from build123d import *

# Parameters (mm, degrees)
SKETCH1_W           = 300
SKETCH1_H           = 500
BOSS_EXTRUDE1_DEPTH = 20
SKETCH1_3_W         = 65
SKETCH1_3_H         = 500
BOSS_EXTRUDE2_DEPTH = 70
CUT_EXTRUDE1_START  = 70
CUT_EXTRUDE1_DEPTH  = 47


with BuildPart() as part:
    # Sketch1 → Boss-Extrude1 (new body)
    with BuildSketch(Plane.XY):
        Rectangle(SKETCH1_W, SKETCH1_H)
    extrude(amount=BOSS_EXTRUDE1_DEPTH)

    # Sketch1<3> → Boss-Extrude2 (add)
    with BuildSketch(Plane.XY):
        with Locations((182.5, 0)):
            Rectangle(SKETCH1_3_W, SKETCH1_3_H)
        with Locations((-182.5, 0)):
            Rectangle(SKETCH1_3_W, SKETCH1_3_H)
    extrude(amount=BOSS_EXTRUDE2_DEPTH)

    # Sketch1<5> → Cut-Extrude1 (cut)
    with BuildSketch(Plane.XY.offset(CUT_EXTRUDE1_START)):
        with BuildLine():
            Line((-164.5, 202.5), (-164.5, -202.5))
            ThreePointArc((-164.5, -202.5), (-182.5, -220.5), (-200.5, -202.5))
            Line((-200.5, -202.5), (-200.5, 202.5))
            ThreePointArc((-200.5, 202.5), (-182.5, 220.5), (-164.5, 202.5))
        make_face()
        with BuildLine():
            Line((164.5, 202.5), (164.5, -202.5))
            ThreePointArc((164.5, -202.5), (182.5, -220.5), (200.5, -202.5))
            Line((200.5, -202.5), (200.5, 202.5))
            ThreePointArc((200.5, 202.5), (182.5, 220.5), (164.5, 202.5))
        make_face()
    extrude(amount=-CUT_EXTRUDE1_DEPTH, mode=Mode.SUBTRACT)


solid = part.part
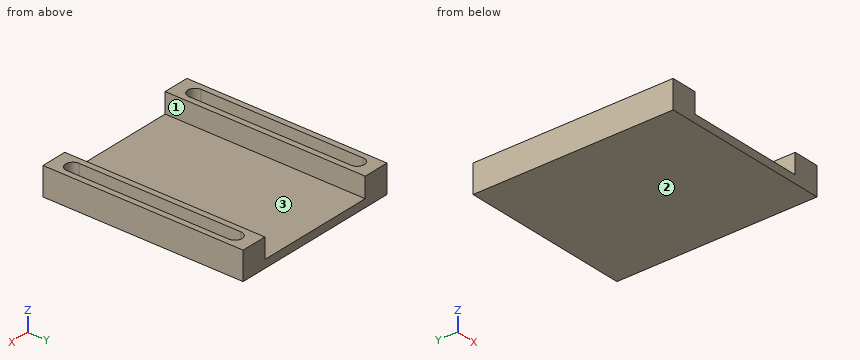
Verification items for the finished model (mm, model axes). Face numbers are marked on the shaded views. Round coordinates to 2 decimals unless told otherwise and drop trailing zeros. Loops run counter-clockwise (first coordinate to the right, second up) from the corner with the lowest first, then second, coordinate; pieces in that order, holes last. Notation, with made-up numbers: (8.5, 28) - (36.5, 28) arc R31 ccw to (36.5, 55) - close; hole circle Ø7 at (-18.75, 88). An arc over 180 degrees is marked (long way). Use a Markdown table: item, result. Add a question column.
1. Section check B-B, the plane x = 182.5. Record the boundary of the cut face in (y, z).
2. Thickness scan on probe 1 along X at (y, z) = (-126, 45); probe 2 along X at (y, z) = (204, 67.5); probe 3 along X at (y, z) = (196.5, 21). Record the ranges inside material, lowest first. Write a range as [from, to].
3. Section check A-A, the plane z = 46.5. Record the boundary of the cut face in (x, y).
4. Section check D-D, the plane x = 38. Record the boundary of the cut face in (y, z).
5. Release check for a two-part mould opening along Z. For the marked faces 1, 2 and 3 record: released by +Z, released by -Z, zero draft, split by the parting line, or undercut.
6. Section check C-C, the plane y = -86.5. Record the boundary of the cut face in (x, z).
7. Gauge pin test, flat ends, axial feed: pin 1 (3 mm diameter, centred on x = -80, y = -184.5, fed in from -Z); pin 2 (18 mm diameter, centred on x = 184, y = 60, fed in from +Z). Record the tip position at first contact, or that the pin passes through.
Checks:
| question | item | result |
|---|---|---|
| 1 | outline | (-250, 0) - (250, 0) - (250, 70) - (220.5, 70) - (220.5, 23) - (-220.5, 23) - (-220.5, 70) - (-250, 70) - close |
| 2 | probe 1 | x = [-215, -200.5], [-164.5, -150], [150, 164.5], [200.5, 215] |
| 2 | probe 2 | x = [-215, -200.44], [-164.56, -150], [150, 164.56], [200.44, 215] |
| 2 | probe 3 | x = [-215, -150], [150, 215] |
| 3 | outline | (-215, -250) - (-150, -250) - (-150, 250) - (-215, 250) - close; (150, -250) - (215, -250) - (215, 250) - (150, 250) - close; hole (-200.5, -202.5) arc R18 ccw to (-164.5, -202.5) - (-164.5, 202.5) arc R18 ccw to (-200.5, 202.5) - close; hole (164.5, -202.5) arc R18 ccw to (200.5, -202.5) - (200.5, 202.5) arc R18 ccw to (164.5, 202.5) - close |
| 4 | outline | (-250, 0) - (250, 0) - (250, 20) - (-250, 20) - close |
| 5 | face 1 | zero draft |
| 5 | face 2 | released by -Z |
| 5 | face 3 | released by +Z |
| 6 | outline | (-215, 0) - (215, 0) - (215, 70) - (200.5, 70) - (200.5, 23) - (164.5, 23) - (164.5, 70) - (150, 70) - (150, 20) - (-150, 20) - (-150, 70) - (-164.5, 70) - (-164.5, 23) - (-200.5, 23) - (-200.5, 70) - (-215, 70) - close |
| 7 | pin 1 | stops at z = 0 |
| 7 | pin 2 | stops at z = 23 |
